from build123d import *

# Parameters (mm, degrees)
ESQUISSE1_W             = 236
ESQUISSE1_H             = 72
BOSS_EXTRU_1_DEPTH      = 3
ENL_V_MAT_EXTRU_1_REACH = 126.314
ESQUISSE2_R             = 2
ESQUISSE3_W             = 236
ESQUISSE3_H             = 6
BOSS_EXTRU_2_DEPTH      = 3


with BuildPart() as part:
    # Esquisse1 → Boss.-Extru.1 (new body)
    with BuildSketch(Plane.XY):
        with Locations((0, -3)):
            Rectangle(ESQUISSE1_W, ESQUISSE1_H)
    extrude(amount=BOSS_EXTRU_1_DEPTH)

    # Esquisse2 → Enlèv. mat.-Extru.1 (cut, up to next)
    with BuildSketch(Plane.XY.offset(3), mode=Mode.PRIVATE) as enl_v_mat_extru_1_sk1:
        with Locations((9, -29)):
            Circle(ESQUISSE2_R)
    enl_v_mat_extru_1_tool1 = extrude(enl_v_mat_extru_1_sk1.sketch, amount=-ENL_V_MAT_EXTRU_1_REACH, mode=Mode.PRIVATE) & part.part
    # Esquisse2 → Enlèv. mat.-Extru.1 (cut, up to next)
    with BuildSketch(Plane.XY.offset(3), mode=Mode.PRIVATE) as enl_v_mat_extru_1_sk2:
        with Locations((-9, -29)):
            Circle(ESQUISSE2_R)
    enl_v_mat_extru_1_tool2 = extrude(enl_v_mat_extru_1_sk2.sketch, amount=-ENL_V_MAT_EXTRU_1_REACH, mode=Mode.PRIVATE) & part.part
    # Esquisse2 → Enlèv. mat.-Extru.1 (cut, up to next)
    with BuildSketch(Plane.XY.offset(3), mode=Mode.PRIVATE) as enl_v_mat_extru_1_sk3:
        with Locations((-9, 23)):
            Circle(ESQUISSE2_R)
    enl_v_mat_extru_1_tool3 = extrude(enl_v_mat_extru_1_sk3.sketch, amount=-ENL_V_MAT_EXTRU_1_REACH, mode=Mode.PRIVATE) & part.part
    # Esquisse2 → Enlèv. mat.-Extru.1 (cut, up to next)
    with BuildSketch(Plane.XY.offset(3), mode=Mode.PRIVATE) as enl_v_mat_extru_1_sk4:
        with Locations((9, 23)):
            Circle(ESQUISSE2_R)
    enl_v_mat_extru_1_tool4 = extrude(enl_v_mat_extru_1_sk4.sketch, amount=-ENL_V_MAT_EXTRU_1_REACH, mode=Mode.PRIVATE) & part.part
    add(enl_v_mat_extru_1_tool1.solids().sort_by_distance((9, -29, 3))[0], mode=Mode.SUBTRACT)
    add(enl_v_mat_extru_1_tool2.solids().sort_by_distance((-9, -29, 3))[0], mode=Mode.SUBTRACT)
    add(enl_v_mat_extru_1_tool3.solids().sort_by_distance((-9, 23, 3))[0], mode=Mode.SUBTRACT)
    add(enl_v_mat_extru_1_tool4.solids().sort_by_distance((9, 23, 3))[0], mode=Mode.SUBTRACT)

    # Esquisse3 → Boss.-Extru.2 (add)
    with BuildSketch(Plane.XY.offset(3)):
        with Locations((0, -42)):
            Rectangle(ESQUISSE3_W, ESQUISSE3_H)
    extrude(amount=-BOSS_EXTRU_2_DEPTH)


solid = part.part
Work out the finished part from the listing and answer in its coordinate system (mm). Give positions to 0.01 mm unless a question says otherwise; leave off trailing zeros. Write each loop counter-clockwise with the first axis right and the second up, starting at its lowest first coordinate (ties: lowest second). Pieces come first, ordered by that corner, then holes. Notation, with made-up numbers: M -6,-13 L 28,-13 A25 cw 28,8 Z; hole C 88,71 d3. An arc over 180 degrees is marked long. Answer as CSV lines item,"result".
Q1. Find the intervals of material crossed by probe 1 along Y at (x, z) = (-9, 2.15); probe 2 along X at (y, z) = (24.5, 1.9), in increasing order. Write a range as [from, to].
A:
probe 1,"y = [-45, -31], [-27, 21], [25, 33]"
probe 2,"x = [-118, -10.32], [-7.68, 7.68], [10.32, 118]"
Q2. A cutting plane is placed at B-B on y = -29. Write down the section's boundary in (x, z), plus the area to 3 significant figures.
A:
outline,"M -118,0 L -11,0 L -11,3 L -118,3 Z; M -7,0 L 7,0 L 7,3 L -7,3 Z; M 11,0 L 118,0 L 118,3 L 11,3 Z"
area,"684 mm²"
Q3. Given P1, Ø6.5, axis at x = -9, y = -29, coming from the -Z side, flat-ended and moving along its own axis, determine where the tip first touches the part or whether it passes through.
A:
P1,"stops at z = 0"
Q4. A cutting plane is placed at A-A on x = 9. Write down the section's boundary in (y, z).
A:
outline,"M -45,0 L -31,0 L -31,3 L -45,3 Z; M -27,0 L 21,0 L 21,3 L -27,3 Z; M 25,0 L 33,0 L 33,3 L 25,3 Z"
Q5. The mould has two halves that part along Y. Classify faces 1 (the flat face through (-2, -5, 0)), 2 (the cylindrical face through (-9, -31, 2)), 3 (the cylindrical face through (7.4, 21.8, 1.5)): +Y half, -Y half, draft (parallel to the pull), parting line (faces both ways), or undercut.
A:
face 1,"draft"
face 2,"undercut"
face 3,"undercut"
